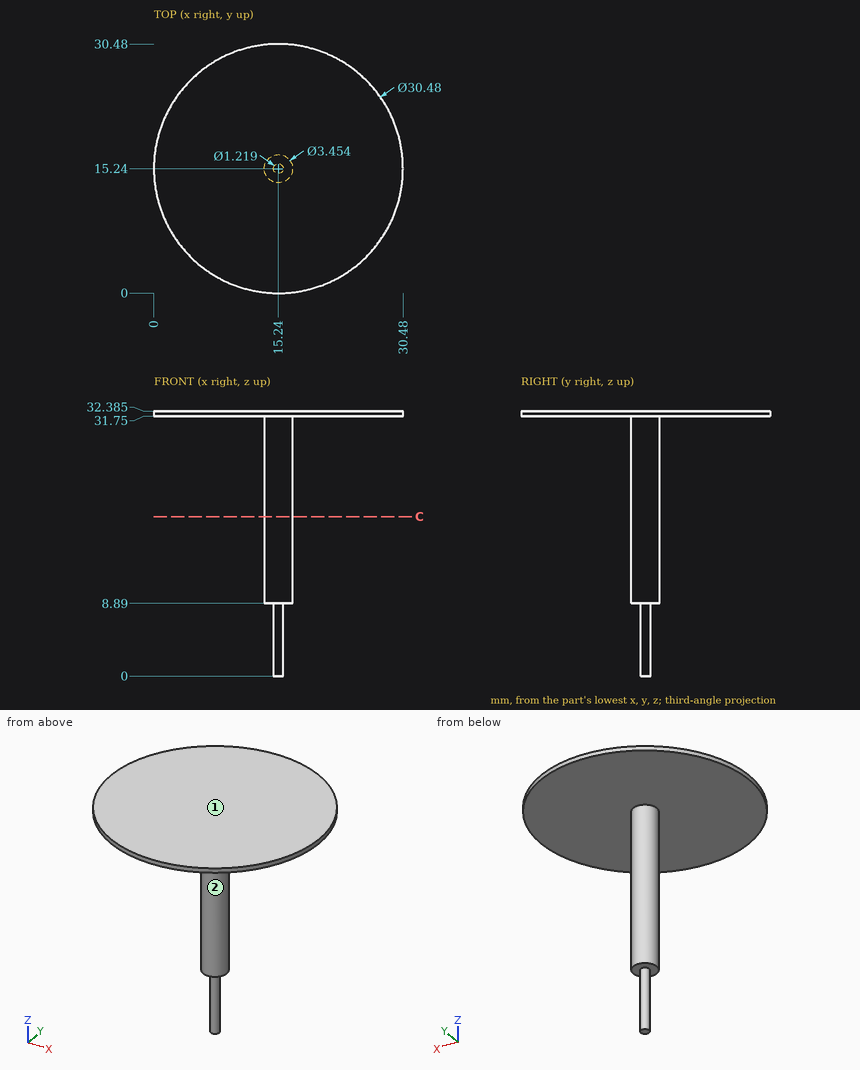
The figure shows three views and two pictorial views of one solid part (mm, origin at its lowest corner). Answer the questions. A direction names the side the tool comes from. Give positions to 0.01 mm unless a question says otherwise; leave off trailing zeros. Order: outer loops, then holes, each group sorted by start corner. A loop starts at its lowest first (then second) coordinate and runs counter-clockwise, first axis right, second up. Notation, with made-up numbers: M -22.5,-3.5 L 22.5,-3.5 A20 ccw 22.5,14.5 Z; hole C 10.5,-36 d1. An arc over 180 degrees is marked long. Return JSON: item names as keys, results as strings.
Q1. Each of these flat-tipped pins is pushed along its axis until it touches: pin 1 (6 mm diameter, centred on x = 25, y = 8, fed in from -Z); pin 2 (12 mm diameter, centred on x = 19.5, z = 5.5, fed in from +Y); pin 3 (10 mm diameter, centred on x = 23.5, z = 3.5, fed in from -Y); pin 4 (6 mm diameter, centred on y = 15.5, z = 28.5, fed in from +X). Where does it stop, or does it pass through?
Answer below:
{"pin 1": "stops at z = 31.75", "pin 2": "stops at y = 16.97", "pin 3": "passes through", "pin 4": "stops at x = 16.97"}
Q2. Which of the six approach directions +Z, -Z, +X, -X, +Y, -Y give full straight-line access (tool end or side, diameter ignored) to the marked faces 1 and 2?
Answer below:
{"face 1": "+Z, +X, -X, +Y, -Y", "face 2": "-Z"}
Q3. Find section C-C, the plane z = 19.5. Write down the section's boundary in (x, y) (1 decimal).
Answer below:
{"outline": "C 15.2,15.2 d3.5"}
Q4. Find the intervals of material crossed by line 1 along Y through (x, z) = (16, 23.5); line 2 along X through (y, z) = (15, 21), in increasing order. Write a range as [from, to].
Answer below:
{"line 1": "y = [13.69, 16.79]", "line 2": "x = [13.53, 16.95]"}
